Could you check a few things on this model? Use its own coordinates, in mm. Round coordinates to 2 decimals unless told otherwise and drop trailing zeros. Order: outer loops, then holes, each group sorted by start corner. A loop starts at its lowest first (then second) coordinate and runs counter-clockwise, first axis right, second up. Notation, with made-up numbers: (27.25, -36) - (45.25, -36) arc R18 ccw to (45.25, -17) - close; hole circle Ø3 at (57.5, 28.5). An arc over 180 degrees is marked (long way). Use one line per item in the form item = value.
from build123d import *

# Parameters (mm, degrees)
BOSS_EXTRUDE1_DEPTH = 10


with BuildPart() as part:
    # Sketch1 → Boss-Extrude1 (new body)
    with BuildSketch(Plane(origin=(0, 0, 0), x_dir=(1, 0, 0), z_dir=(0, 1, 0))):
        with BuildLine():
            Line((0, 120), (0, 60))
            Line((0, 60), (15, 60))
            ThreePointArc((15, 60), (20, 65), (25, 60))
            Line((25, 60), (40, 60))
            Line((40, 60), (40, 120))
            Line((40, 120), (0, 120))
        make_face()
        with BuildLine():
            Line((0, 60), (0, 0))
            Line((0, 0), (40, 0))
            Line((40, 0), (40, 60))
            Line((40, 60), (25, 60))
            ThreePointArc((25, 60), (20, 55), (15, 60))
            Line((15, 60), (0, 60))
        make_face()
    extrude(amount=BOSS_EXTRUDE1_DEPTH)


solid = part.part
Item 1: Will this pin go through, and if not, where does the flat tip stop? P1, Ø6, axis at x = 20, z = -60, coming from the +Y side.
Found:
P1 = through
Item 2: If we mould it in two halves opening along Z, with no side actions, what happens to faces 1 (the face through (20, 5, 0)), 2 (the face through (19.349, 4.93, -55.043)), 3 (the face through (40, 5, -59))? For each: released by +Z, released by -Z, zero draft, split by the parting line, or undercut.
Found:
face_1 = released by +Z
face_2 = undercut
face_3 = zero draft
Item 3: I need wall thicknesses on L1, parallel to Z at x = 20, y = 4; L2, parallel to Z at x = 22, y = 5.25; L3, parallel to X at y = 3.5, z = -57. Which ranges of each line are inside material? Lowest first, please.
Found:
L1 = -120 to -65, -55 to 0
L2 = -120 to -64.58, -55.42 to 0
L3 = 0 to 16, 24 to 40
Item 4: Imagine slicing it at C-C on x = 20. Please give me the cut outline in (y, z).
Found:
outline = (0, -120) - (10, -120) - (10, -65) - (0, -65) - close; (0, -55) - (10, -55) - (10, 0) - (0, 0) - close
Item 5: Imagine slicing it at B-B on y = 6.5. Please give me the cut outline in (x, z), plus the area to 3 significant figures.
Found:
outline = (0, -120) - (40, -120) - (40, 0) - (0, 0) - close; hole circle Ø10 at (20, -60)
area = 4,720 mm2
Item 6: Imagine slicing it at A-A on z = -60. Please give me the cut outline in (x, y), plus the area to 3 significant figures.
Found:
outline = (0, 0) - (15, 0) - (15, 10) - (0, 10) - close; (25, 0) - (40, 0) - (40, 10) - (25, 10) - close
area = 300 mm2
